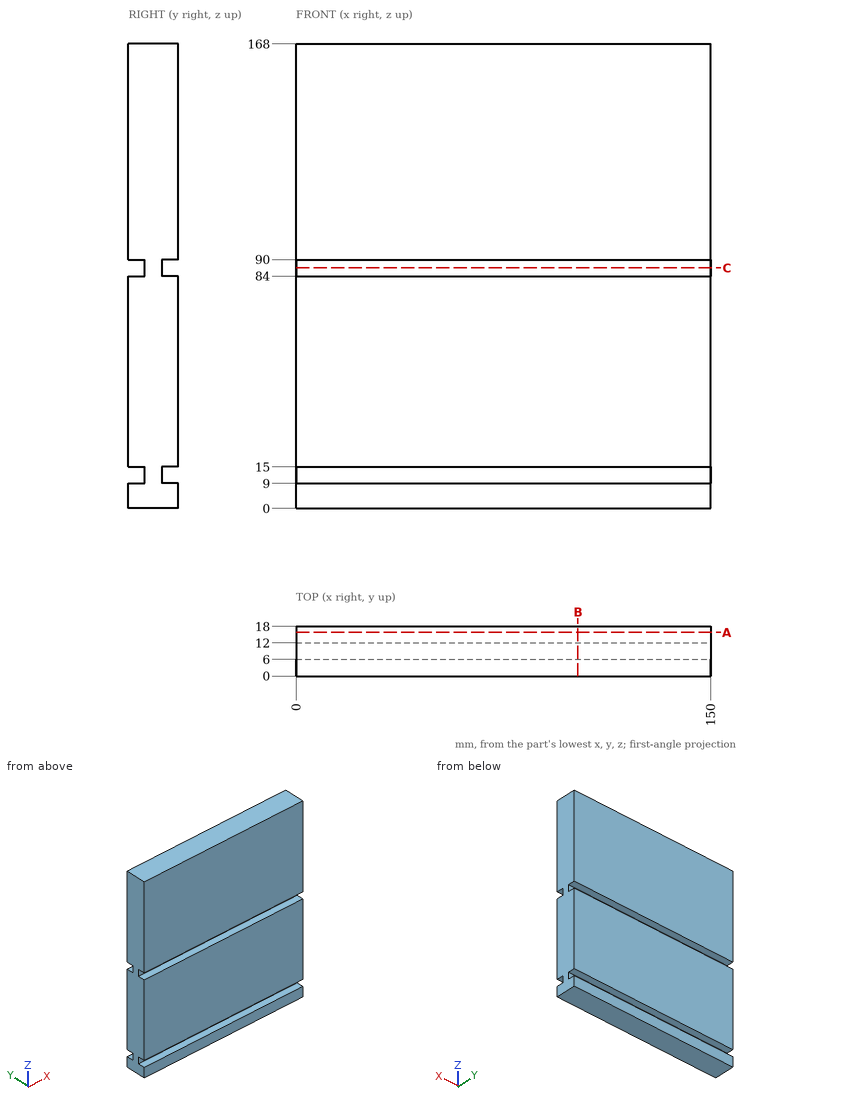
Here's the drawing with two shaded views (mm, measured from the low corner). I have some questions. Give positions to 0.01 mm unless a question says otherwise; leave off trailing zeros. Loops run counter-clockwise (first coordinate to the right, second up) from the corner with the lowest first, then second, coordinate; pieces in that order, holes last. Notation, with made-up numbers: M 4.5,-1 L 45.5,-1 A31 cw 45.5,38 Z; hole C -0.5,-39.5 d8. An arc over 180 degrees is marked long. Use one line per item in the form item = value. Start each with the question number.
Q1. I need wall thicknesses on line 1 along Z through (x, y) = (31.5, 13.25). Which ranges of the line are inside material? Lowest first, please.
Q2. Will these pins go through, and if not, where does the flat tip stop? pin 1 Ø2 at (x, z) = (78, 57.5) entering from -Y; pin 2 Ø3 at (x, z) = (54, 86) entering from -Y; pin 3 Ø3 at (x, z) = (108.5, 11) entering from +Y.
Q3. If we section it at C-C (z = 87): Write out the boundary of the cut face in (x, y).
Q4. If we section it at B-B (x = 102): Write out the boundary of the cut face in (y, z), then the cut area to 3 significant figures.
Q5. If we section it at A-A (y = 15.75): Write out the boundary of the cut face in (x, z), then the cut area to 3 significant figures.
Taken from the geometry:
q1.line_1 = 0 to 9, 15 to 84, 90 to 168
q2.pin_1 = 0
q2.pin_2 = 6
q2.pin_3 = 12
q3.outline = M 0,6 L 150,6 L 150,12 L 0,12 Z
q4.outline = M 0,0 L 18,0 L 18,9 L 12,9 L 12,15 L 18,15 L 18,84 L 12,84 L 12,90 L 18,90 L 18,168 L 0,168 L 0,90 L 6,90 L 6,84 L 0,84 L 0,15 L 6,15 L 6,9 L 0,9 Z
q4.area = 2,880 mm^2
q5.outline = M 0,0 L 150,0 L 150,9 L 0,9 Z; M 0,15 L 150,15 L 150,84 L 0,84 Z; M 0,90 L 150,90 L 150,168 L 0,168 Z
q5.area = 23,400 mm^2
